The listing builds one solid part. Answer for the finished solid, in the listing's coordinates (mm). A direction names the side the tool comes from. Coordinates: 2 decimals unless noted, no trailing zeros. Loops run counter-clockwise (first coordinate to the right, second up) from the corner with the lowest first, then second, coordinate; pieces in that order, holes last. Notation, with made-up numbers: M 52.5,32 L 107.5,32 A19 cw 107.5,48 Z; hole C 3,-39 d4. An arc over 180 degrees is marked long. Answer as a JSON object with one key per item and string values. Group by question number.
1. Given pin 1 (5.5 mm diameter, centred on x = 8.5, z = 0, fed in from -Y); pin 2 (3 mm diameter, centred on x = -19, z = -0.5, fed in from +Y); pin 3 (0.8 mm diameter, centred on x = -19.5, z = 1, fed in from -Y); pin 4 (0.8 mm diameter, centred on y = -16.5, z = -0.5, fed in from -X), each flat-ended and moving along its own axis, determine where each tip first touches the part or whether it passes through.
2. A cutting plane is placed at B-B on y = -9. Give the vertices of the cut face in (x, z), and give its area (3 significant figures).
3. Determine the mould class of faces 5 (the face through (-4, 0, 5.08)), 6 (the face through (17, 0, -2.54)), 7 (the face through (0, -17.78, 3)) for opening direction Y: released by +Y, released by -Y, zero draft, split by the parting line, or undercut.
4. Straight lines are drawn through the part: L1, parallel to X at y = -7, z = 1.25; L2, parallel to Y at x = -9, z = 3.5; L3, parallel to X at y = 1.5, z = 1.5. For each, find the intervals that lie inside material, in ascending order.
5. A cutting plane is placed at A-A on x = -3. Give the vertices of the cut face in (y, z), and give its area (3 significant figures).
6. A cutting plane is placed at C-C on y = -14. Give the vertices of the cut face in (x, z), and give its area (3 significant figures).
7. For faces 1 (the face through (-19, 9.906, 0)), 2 (the face through (-19, 0, 2.286)), 3 (the face through (1.398, 3.186, 0.071)), 4 (the face through (-19, -9.906, 0)), determine the directions among +Z, -Z, +X, -X, +Y, -Y from which every point of the face is accessible in a straight line to the end or side of a thin tool.
from build123d import *

# Parameters (mm, degrees)
F0_W     = 35.56
F0_H     = 35.56
F1_DEPTH = 5.08
F2_W     = 19.812
F2_H     = 4.572
F3_DEPTH = 2.54
F4_W     = 19.812
F4_H     = 4.572
F5_DEPTH = 2.54
F6_W     = 20.32
F6_H     = 5.08
F7_DEPTH = 2.54
F8_W     = 20.32
F8_H     = 5.08
F9_DEPTH = 2.54


with BuildPart() as f1:
    # F0 (on Top) → F1 (new body, symmetric)
    with BuildSketch(Plane.XY):
        Rectangle(F0_W, F0_H)
        with BuildLine():
            Line((11.6113498264, 12.4850260417), (11.6113498264, -12.7))
            Line((11.6113498264, -12.7), (4.8258897569, -12.7))
            Line((4.8258897569, -12.7), (-6.1322699653, 6.35))
            Line((-6.1322699653, 6.35), (-6.2866102431, 6.35))
            add(Edge.make_bspline(
                [(-6.2866102431, 6.35), (-5.9558810764, 1.3063802083), (-5.9558810764, -0.8488715278)],
                knots=[0, 0, 0, 1, 1, 1], degree=2))
            Line((-5.9558810764, -0.8488715278), (-5.9558810764, -12.7))
            Line((-5.9558810764, -12.7), (-10.7294053819, -12.7))
            Line((-10.7294053819, -12.7), (-10.7294053819, 12.4850260417))
            Line((-10.7294053819, 12.4850260417), (-3.9935546875, 12.4850260417))
            Line((-3.9935546875, 12.4850260417), (6.9425564236, -6.3775607639))
            Line((6.9425564236, -6.3775607639), (7.0638237847, -6.3775607639))
            add(Edge.make_bspline(
                [(7.0638237847, -6.3775607639), (6.8047526042, -1.4662326389), (6.8047526042, 0.5622395833)],
                knots=[0, 0, 0, 1, 1, 1], degree=2))
            Line((6.8047526042, 0.5622395833), (6.8047526042, 12.4850260417))
            Line((6.8047526042, 12.4850260417), (11.6113498264, 12.4850260417))
        make_face(mode=Mode.SUBTRACT)
    extrude(amount=F1_DEPTH, both=True)

    # F2 (on face) → F3 (join)
    with BuildSketch(Plane(origin=(0, 17.78, 0), x_dir=(-1, 0, 0), z_dir=(0, 1, 0))):
        Rectangle(F2_W, F2_H)
    extrude(amount=F3_DEPTH)

    # F4 (on face) → F5 (join)
    with BuildSketch(Plane(origin=(-17.78, 0, 0), x_dir=(0, -1, 0), z_dir=(-1, 0, 0))):
        Rectangle(F4_W, F4_H)
    extrude(amount=F5_DEPTH)

    # F6 (on face) → F7 (cut)
    with BuildSketch(Plane.XZ.offset(17.78)):
        Rectangle(F6_W, F6_H)
    extrude(amount=-F7_DEPTH, mode=Mode.SUBTRACT)

    # F8 (on face) → F9 (cut)
    with BuildSketch(Plane.YZ.offset(17.78)):
        Rectangle(F8_W, F8_H)
    extrude(amount=-F9_DEPTH, mode=Mode.SUBTRACT)


solid = f1.part
From the geometry:
{
 "1": {"pin 1": "stops at y = -17.78", "pin 2": "stops at y = 17.78", "pin 3": "stops at y = -9.91", "pin 4": "stops at x = -17.78"},
 "2": {"outline": "M -20.32,-2.29 L -17.78,-2.29 L -17.78,-5.08 L -10.73,-5.08 L -10.73,5.08 L -17.78,5.08 L -17.78,2.29 L -20.32,2.29 Z; M -5.96,-5.08 L 2.7,-5.08 L 2.7,5.08 L -5.96,5.08 Z; M 11.61,-5.08 L 17.78,-5.08 L 17.78,-2.54 L 15.24,-2.54 L 15.24,2.54 L 17.78,2.54 L 17.78,5.08 L 11.61,5.08 Z", "area": "221 mm²"},
 "3": {"face 5": "zero draft", "face 6": "undercut", "face 7": "released by -Y"},
 "4": {"L1": "x = -20.32 to -10.73, -5.96 to 1.55, 11.61 to 15.24", "L2": "y = -17.78 to -12.7, 12.49 to 17.78", "L3": "x = -20.32 to -10.73, -6.02 to -3.34, 2.38 to 6.8, 11.61 to 15.24"},
 "5": {"outline": "M -17.78,-5.08 L 0.9,-5.08 L 0.9,5.08 L -17.78,5.08 L -17.78,2.54 L -15.24,2.54 L -15.24,-2.54 L -17.78,-2.54 Z; M 10.77,-5.08 L 17.78,-5.08 L 17.78,-2.29 L 20.32,-2.29 L 20.32,2.29 L 17.78,2.29 L 17.78,5.08 L 10.77,5.08 Z", "area": "260 mm²"},
 "6": {"outline": "M -17.78,-5.08 L 17.78,-5.08 L 17.78,5.08 L -17.78,5.08 Z", "area": "361 mm²"},
 "7": {"face 1": "+Z, -Z, -X, +Y", "face 2": "+Z, -X, +Y, -Y", "face 3": "+Z, -Z", "face 4": "+Z, -Z, -X, -Y"}
}
